Geometry: see drawing. Coordinates: mm, zero at the bounding-box minimum. A direction names the side the tool comes from. Give positions to 0.01 mm unless a question says otherwise; leave off trailing zeros. Write each loop counter-clockwise with the first axis right and the second up, starting at its lowest first coordinate (ties: lowest second). Pieces come first, ordered by that corner, then holes. Notation, with made-up numbers: M 59.5,57 L 114.5,57 A21 cw 114.5,89 Z; hole C 18,9.5 d6. An arc over 180 degrees is marked long. Use one line per item in the form item = value. Start each with the question number.
Item 1: Material intervals for line 1 along Z through (x, y) = (84, 4) (1 decimal), sorted ascending. Write a range as from..to.
Item 2: Access query for the marked faces 1 and 2. Directions: +Z, -Z, +X, -X, +Y, -Y. A direction counts if a zero-diameter tool reaches every point of the face in a straight line with its end or side. Return the directions, or none.
Item 3: Section query D-D on y = 48.5. Return loops of the section in (x, z) (1 decimal).
Item 4: Section query A-A on x = 26. Return loops of the section in (y, z) (1 decimal).
Item 5: Contact query for a flat-ended pin moving along its axis: P1, Ø9, axis at x = 62.76, y = 11.43, coming from the -Z side (3 decimals). Output: stop coordinate, or through.
Item 6: Section query B-B on z = 38. Return loops of the section in (x, y) (1 decimal).
Item 7: Section query C-C on y = 11.43. Return loops of the section in (x, z) (1 decimal), then the cut area to 3 significant figures.
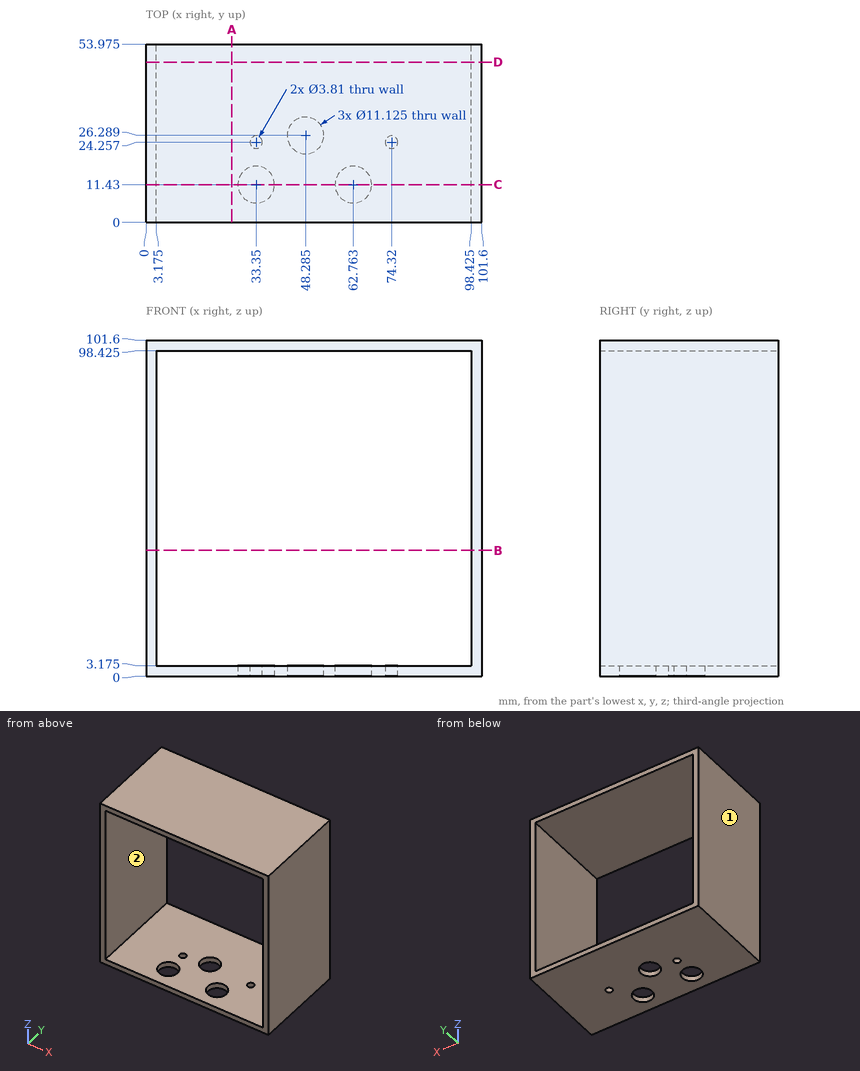
Answer sheet:
q1.line_1 = 0..3.2, 98.4..101.6
q2.face_1 = +Z, -Z, -X, +Y, -Y
q2.face_2 = +Y, -Y
q3.outline = M 0,0 L 101.6,0 L 101.6,101.6 L 0,101.6 Z; hole M 3.2,3.2 L 98.4,3.2 L 98.4,98.4 L 3.2,98.4 Z
q4.outline = M 0,0 L 54,0 L 54,3.2 L 0,3.2 Z; M 0,98.4 L 54,98.4 L 54,101.6 L 0,101.6 Z
q5.P1 = 98.425
q6.outline = M 0,0 L 3.2,0 L 3.2,54 L 0,54 Z; M 98.4,0 L 101.6,0 L 101.6,54 L 98.4,54 Z
q7.outline = M 0,0 L 27.8,0 L 27.8,3.2 L 3.2,3.2 L 3.2,98.4 L 98.4,98.4 L 98.4,3.2 L 68.3,3.2 L 68.3,0 L 101.6,0 L 101.6,101.6 L 0,101.6 Z; M 38.9,0 L 57.2,0 L 57.2,3.2 L 38.9,3.2 Z
q7.area = 1,180 mm2
